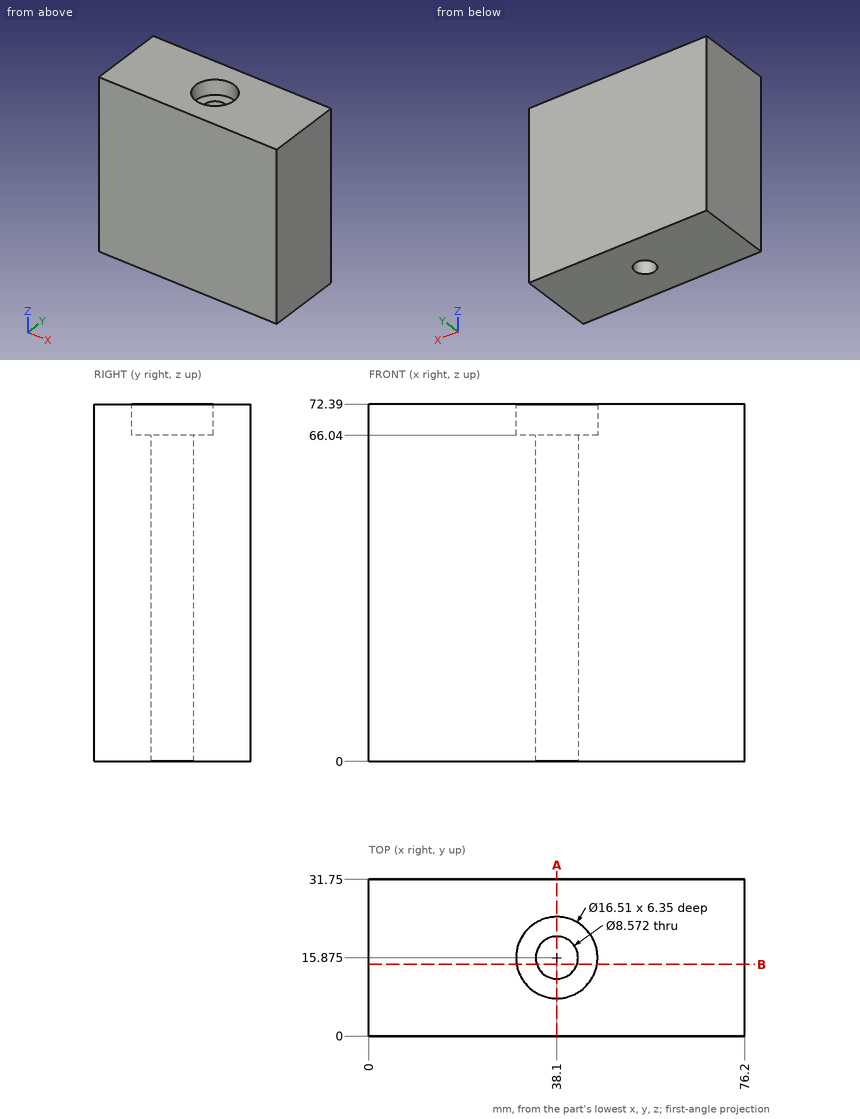
Input: dimensioned drawing with shaded views. Units: mm. Origin: part minimum x, y, z. Round coordinates to 2 decimals unless told otherwise and drop trailing zeros. Order: outer loops, then holes, each group sorted by start corner. A loop starts at its lowest first (then second) coordinate and runs counter-clockwise, first axis right, second up.
1. Material intervals for line 1 (X direction, y = 15.5, z = 35.5); line 2 (Y direction, x = 38.1, z = 68.25); line 3 (X direction, y = 15, z = 60) (1 decimal), sorted ascending.
The answers:
line 1: x = 0 to 33.83, 42.37 to 76.2
line 2: y = 0 to 7.62, 24.13 to 31.75
line 3: x = 0 to 33.9, 42.3 to 76.2
2. Cut plane B-B, the plane y = 14.5. Output: boundary loops of the cut face in (x, z).
The answers:
outline: (0, 0) - (34.04, 0) - (34.04, 66.04) - (29.96, 66.04) - (29.96, 72.39) - (0, 72.39) - close; (42.16, 0) - (76.2, 0) - (76.2, 72.39) - (46.24, 72.39) - (46.24, 66.04) - (42.16, 66.04) - close
3. Cut plane A-A, the plane x = 38.1. Output: boundary loops of the cut face in (y, z), then the cut area to 3 significant figures.
The answers:
outline: (0, 0) - (11.59, 0) - (11.59, 66.04) - (7.62, 66.04) - (7.62, 72.39) - (0, 72.39) - close; (20.16, 0) - (31.75, 0) - (31.75, 72.39) - (24.13, 72.39) - (24.13, 66.04) - (20.16, 66.04) - close
area: 1,630 mm2
